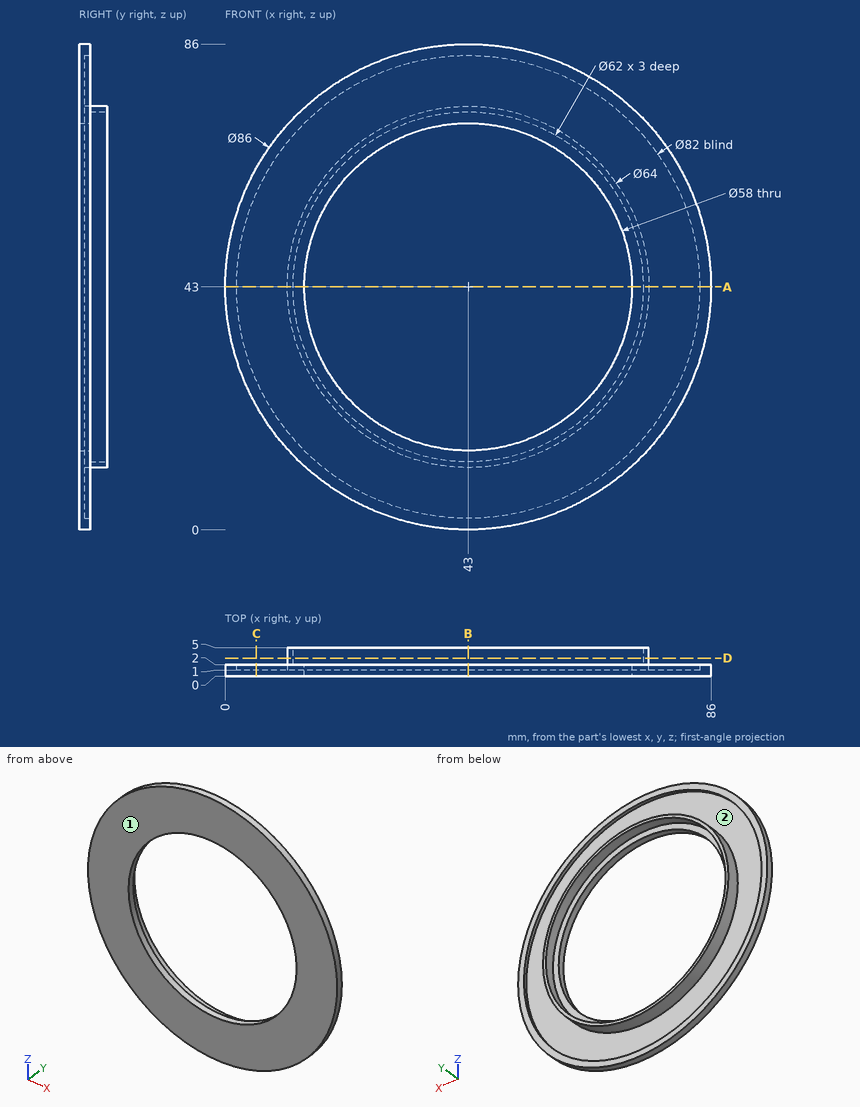
Geometry check sheet. Reference: drawing and pictorial views, mm from the part's lowest x, y, z. Round coordinates to 2 decimals unless told otherwise and drop trailing zeros. Write each loop counter-clockwise with the first axis right and the second up, starting at its lowest first coordinate (ties: lowest second). Pieces come first, ordered by that corner, then holes. Notation, with made-up numbers: (50, -39.5) -> (105, -39.5) arc R17 cw to (105, -19.5) -> close; hole circle Ø1 at (-5, -13). An arc over 180 degrees is marked (long way). Put each result on its own line as item: value.
1) Cross-section at D-D, the plane y = 3.15. Enter the section's corners in (x, z).
Recorded:
outline: circle Ø64 at (43, 43); hole circle Ø62 at (43, 43)
2) Thickness scan on probe 1 along Z at (x, y) = (43, 1.65); probe 2 along X at (y, z) = (1.3, 39). Record the ranges inside material, lowest first. Write a range as from..to.
Recorded:
probe 1: z = 0..2, 11..14, 72..75, 84..86
probe 2: x = 0.19..2.2, 11.25..14.28, 71.72..74.75, 83.8..85.81
3) Cross-section at C-C, the plane x = 5.5. Enter the section's corners in (y, z).
Recorded:
outline: (0, 21.96) -> (2, 21.96) -> (2, 26.42) -> (1, 26.42) -> (1, 59.58) -> (2, 59.58) -> (2, 64.04) -> (0, 64.04) -> close
4) Depth check by flat-ended pin: P1, Ø18.5, axis at x = 30, z = 55, coming from the +Y side. Enter the tip coordinate at first touch or a pass-through.
Recorded:
P1: passes through
5) Cross-section at B-B, the plane x = 43. Enter the section's corners in (y, z), plus the area to 3 significant figures.
Recorded:
outline: (0, 0) -> (2, 0) -> (2, 2) -> (1, 2) -> (1, 11) -> (5, 11) -> (5, 12) -> (2, 12) -> (2, 14) -> (0, 14) -> close; (0, 72) -> (2, 72) -> (2, 74) -> (5, 74) -> (5, 75) -> (1, 75) -> (1, 84) -> (2, 84) -> (2, 86) -> (0, 86) -> close
area: 44.0 mm2
6) Release check for a two-part mould opening along X. For the marked faces 1 and 2 record: pulls with the +X half, pulls with the -X half, needs draft (parallel to the pull), parting line crosses it, or undercut.
Recorded:
face 1: needs draft
face 2: undercut
7) Cross-section at A-A, the plane z = 43. Enter the section's corners in (x, y).
Recorded:
outline: (0, 0) -> (14, 0) -> (14, 2) -> (12, 2) -> (12, 5) -> (11, 5) -> (11, 1) -> (2, 1) -> (2, 2) -> (0, 2) -> close; (72, 0) -> (86, 0) -> (86, 2) -> (84, 2) -> (84, 1) -> (75, 1) -> (75, 5) -> (74, 5) -> (74, 2) -> (72, 2) -> close
